Can you work these out from the model? Positions are in its coordinate system, mm. Face numbers are marked on the shaded views. A direction names the side the tool comes from. Give positions to 0.01 mm unless a question says otherwise; leave off trailing zeros. Write each loop counter-clockwise with the first axis right and the second up, starting at its lowest first coordinate (ties: lowest second). Pieces come first, ordered by that corner, then holes.
1. I'm going to push flat-ended pins straight in: pin 1 (4 mm diameter, centred on x = 215.5, z = -201, fed in from +Y); pin 2 (15 mm diameter, centred on x = 138.5, z = -123.5, fed in from +Y); pin 3 (4 mm diameter, centred on x = 149.5, y = 10, fed in from -Z); pin 4 (14.5 mm diameter, centred on x = 280.66, z = -260.34, fed in from -Y). Where does each tip first touch, or does it pass through?
2. If I drill on probe 1 along Z at (x, y) = (303, 29); probe 2 along Z at (x, y) = (373, 12); probe 3 along X at (y, z) = (5.5, -312), over which ranges is the centre line in solid material (lowest first)?
3. Suppose I cut it at D-D (x = 303.4). Please give me the cut outline in (y, z).
4. Suppose I cut it at A-A (x = 373). Please give me the cut outline in (y, z), and give its area (3 significant figures).
5. Suppose I cut it at C-C (z = -11). Please give me the cut outline in (x, y), and give its area (3 significant figures).
6. Thinking about a two-plate mould opening in X: for the marked faces 6, 7 and 8, which applies, pulls with the +X half, pulls with the -X half, needs draft (parallel to the pull), parting line crosses it, or undercut?
7. On a 3-axis mill with a long thin cutter (end or side, diameter ignored), from which of +Z, -Z, +X, -X, +Y, -Y can I reach the whole of each face in a straight line? I mean the marked faces 1, 2, 3, 4 and 5. Say none if no direction works.
8. Suppose I cut it at B-B (z = -274). Please give me the cut outline in (x, y).
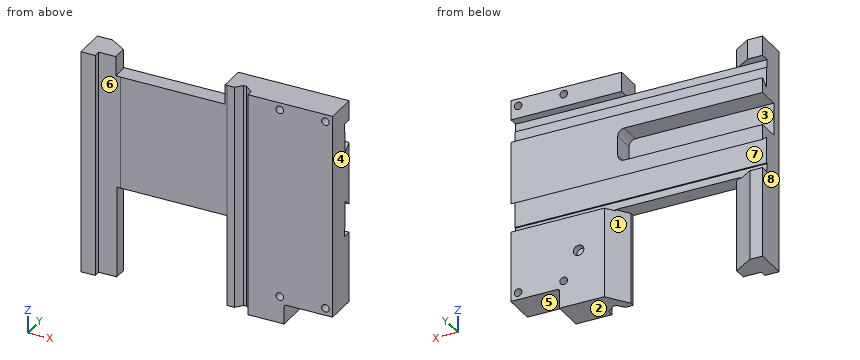
Autodesk Inventor part; units mm, degrees
ref_plane "YZ Plane" through (0, 0, 0) normal (1, 0, 0) x (0, 1, 0)
ref_plane "XZ Plane" through (0, 0, 0) normal (0, 1, 0) x (-1, 0, 0)
ref_plane "XY Plane" through (0, 0, 0) normal (0, 0, 1) x (1, 0, 0)
sketch "Sketch1" plane through (0, 0, 0) normal (0, 1, 0) x (-1, 0, 0)
  line L0 (0, 0) -> (-384, 0)
  line L1 (-384, 0) -> (-384, -343)
  line L2 (-384, -343) -> (0, -343)
  line L3 (0, -343) -> (0, 0)
  dimension "d0" = 384
  dimension "d1" = 343
extrude "Extrusion1" add sketch "Sketch1" along normal blind 48.5
sketch "Sketch3" plane through (384, 0, 0) normal (1, 0, 0) x (0, 0, -1)
  line L0 (0, 0) -> (343, 0)
  line L1 (0, 0) -> (0, 48.5)
  line L2 (343, 0) -> (343, 48.5)
  line L3 (30, 48.5) -> (65, 48.5)
  line L4 (30, 48.5) -> (30, 37)
  line L5 (65, 48.5) -> (74.6496, 37)
  line L6 (43, 37) -> (74.6496, 37)
  line L7 (30, 37) -> (30, 35)
  line L8 (30, 35) -> (43, 35)
  line L9 (43, 35) -> (43, 37)
  dimension "d23" = 35
  dimension "d37" = 2
  dimension "d38" = 13
extrude "Extrusion2" cut sketch "Sketch3" against normal through all
sketch "Sketch7" plane through (384, 0, 0) normal (1, 0, 0) x (0, 0, -1)
  line L0 (65, 48.5) -> (343, 48.5)
  line L1 (65, 48.5) -> (161, 48.5)
  line L2 (161, 48.5) -> (174.2196, 48.5) construction
  line L3 (161, 48.5) -> (205, 48.5)
  line L4 (0, 0) -> (343, 0)
  line L5 (151.3504, 37) -> (192, 37)
  line L6 (205, 37) -> (205, 48.5)
  line L7 (161, 48.5) -> (151.3504, 37)
  line L8 (161, 48.5) -> (183.0653, 48.5) construction
  line L9 (205, 37) -> (205, 35)
  line L10 (205, 35) -> (192, 35)
  line L11 (192, 35) -> (192, 37)
  dimension "d27" = 96
  dimension "d29" = 44
  dimension "d32" = 130
extrude "Extrusion3" cut sketch "Sketch7" against normal through all
sketch "Sketch8" plane through (0, 48.5, 0) normal (0, 1, 0) x (1, 0, 0)
  line L0 (310, 343) -> (310, 316)
  line L1 (313, 313) -> (384, 313)
  line L2 (384, 0) -> (384, 343)
  line L3 (384, 313) -> (384, 343)
  line L4 (384, 343) -> (310, 343)
  line L5 (384, 343) -> (0, 343)
  arc A0 (310, 316) -> (313, 313) centre (313, 316) ccw
  point P0 (0, 0)
  point P1 (310, 313)
  dimension "d43" = 30
  dimension "d46" = 3
extrude "Extrusion4" cut sketch "Sketch8" against normal through all
sketch "Sketch12" plane through (0, 48.5, 0) normal (0, 1, 0) x (1, 0, 0)
  line L0 (221, 113) -> (221, 128)
  line L1 (211, 88) -> (0, 88)
  line L2 (211, 138) -> (0, 138)
  arc A0 (211, 88) -> (221, 98) centre (211, 98) ccw
  arc A1 (221, 128) -> (211, 138) centre (211, 128) ccw
  line L3 (221, 98) -> (221, 113)
  line L4 (0, 88) -> (0, 138)
  point P0 (384, 161)
  point P1 (221, 88)
  dimension "d72" = 10
extrude "Extrusion8" cut sketch "Sketch12" against normal blind 33
sketch "Sketch28" plane through (0, 48.5, 0) normal (0, 1, 0) x (1, 0, 0)
  circle A0 centre (373, 302) radius 5.8
  circle A1 centre (303.4, 302) radius 5.8
  circle A2 centre (373, 11) radius 5.8
  circle A3 centre (303.4, 11) radius 5.8
  point P0 (0, 0)
  point P1 (384, 313)
  point P2 (384, 0)
  dimension "d146" = 11.6
  dimension "d149" = 11.6
  dimension "d152" = 11.6
  dimension "d155" = 11.6
extrude "Extrusion19" cut sketch "Sketch28" against normal through all
sketch "Sketch29" plane through (0, 48.5, 0) normal (0, 0, 1) x (1, 0, 0)
  line L0 (0, -48.5) -> (0, 0)
  line L1 (0, 0) -> (384, 0)
  line L2 (23, 0) -> (48, -16.2352)
  line L3 (23, 0) -> (48, -16.2352)
  line L4 (0, -48.5) -> (384, -48.5)
  line L5 (23, 0) -> (48, 0)
  line L6 (48, -16.2352) -> (48, 0)
  line L7 (384, -13.5) -> (0, -13.5)
  point P0 (48, -48.5)
  point P1 (215, -48.5)
  point P2 (20, -48.5)
extrude "Extrusion20" cut sketch "Sketch29" against normal up to surface (30 mm away) contours L7 L6 L2 | L2 L1 L6 L7
sketch "Sketch30" plane through (0, 0, 0) normal (0, 0, 1) x (1, 0, 0)
  line L0 (48, 48.5) -> (215, 48.5)
  line L1 (215, 48.5) -> (215, 0)
  line L2 (215, 0) -> (48, 0)
  line L3 (48, 0) -> (48, 48.5)
  point P0 (0, 0)
  point P1 (48, 0)
extrude "Extrusion21" cut sketch "Sketch30" against normal up to surface (30 mm away)
sketch "Sketch32" plane through (0, 48.5, 0) normal (0, 1, 0) x (1, 0, 0)
  line L0 (275, 266) -> (283, 266) construction
  circle A0 centre (280.6569, 260.3431) radius 8
  point P0 (0, 0)
  point P1 (255, 343)
  dimension "d168" = 16
extrude "Extrusion22" cut sketch "Sketch32" against normal blind 10
sketch "Sketch36" plane through (0, 0, -343) normal (0, 0, -1) x (-1, 0, 0)
  line L0 (-255, 0) -> (-243.6863, 11.3137)
  line L1 (-255, 0) -> (-239, 0) construction
  line L2 (-243.6863, 11.3137) -> (-239.0863, 11.3137)
  line L3 (-239.0863, 11.3137) -> (-229.7525, 1.9799)
  line L4 (-239.0863, 11.3137) -> (-225.8863, 11.3137) construction
  line L5 (-229.7525, 1.9799) -> (-217.7525, 1.9799)
  line L6 (-22, 0) -> (-22, 10)
  line L7 (-22, 10) -> (-55, 10)
  line L8 (-217.7525, 1.9799) -> (-217.7525, 0)
  line L9 (-55, 10) -> (-55, 0)
  line L10 (-255, 0) -> (-217.7525, 0)
  line L11 (-310, 0) -> (0, 0)
  line L12 (-55, 0) -> (-22, 0)
  dimension "d209" = 16
  dimension "d210" = 45
  dimension "d211" = 4.6
  dimension "d214" = 13.2
  dimension "d215" = 45
  dimension "d216" = 12
  dimension "d224" = 22
  dimension "d225" = 10
extrude "Extrusion23" cut sketch "Sketch36" against normal through all
sketch "Sketch37" plane through (0, 0, -343) normal (0, 0, -1) x (-1, 0, 0)
  line L0 (-217.7525, 1.9799) -> (-217.7525, 15.9799)
  line L1 (-217.7525, 15.9799) -> (-241.3863, 48.5)
  line L2 (-241.3863, 48.5) -> (-19.5919, 48.5)
  line L3 (-211, 48.5) -> (0, 48.5)
  line L4 (-48, 10) -> (-55, 10)
  line L5 (-217.7525, 0) -> (-217.7525, 1.9799)
  line L6 (-217.7525, 1.9799) -> (-217.7525, 0)
  line L7 (-215, 0) -> (-55, 0)
  line L8 (-217.7525, 0) -> (-55, 0)
  line L9 (-55, 10) -> (-55, 0)
  line L10 (-55, 0) -> (-55, 10)
  line L11 (-217.7525, 15.9799) -> (-49.7525, 15.9799) construction
  line L12 (-55, 10) -> (-49.7525, 10)
  line L13 (-49.7525, 10) -> (-49.7525, 29)
  line L14 (-49.7525, 29) -> (-19.5919, 48.5)
  line L15 (0, 48.5) -> (-23, 48.5)
  point P0 (0, 0)
  dimension "d229" = 14
  dimension "d232" = 19
extrude "Extrusion24" cut sketch "Sketch37" against normal blind 140
sketch "Sketch38" plane through (0, 0, -203) normal (0, 0, -1) x (-1, 0, 0)
  line L0 (-49.7525, 29) -> (-49.7525, 10)
  line L1 (-55, 9.9841) -> (-217.7525, 9.4921)
  line L2 (-217.7525, 1.9799) -> (-217.7525, 15.9799)
  line L3 (-217.7525, 0) -> (-217.7525, 1.9799)
  line L4 (-217.7525, 9.4921) -> (-217.7525, 0)
  line L5 (-215, 0) -> (-55, 0)
  line L6 (-217.7525, 0) -> (-55, 0)
  line L7 (-55, 10) -> (-55, 0)
  line L8 (-55, 0) -> (-55, 10)
  line L9 (-55, 10) -> (-55, 0)
  point P0 (0, 0)
extrude "Extrusion25" cut sketch "Sketch38" against normal through all
sketch "Sketch40" plane through (0, 0, -343) normal (0, 0, -1) x (-1, 0, 0)
  line L0 (-229.5482, 9.4921) -> (-238.1559, 19.4995)
  line L1 (-229.5482, 9.4921) -> (-216.3482, 9.4921) construction
  line L2 (-238.1559, 19.4995) -> (-242.7559, 19.4995)
  line L3 (-242.7559, 19.4995) -> (-255, 9.1999)
  line L4 (-242.7559, 19.4995) -> (-226.7559, 19.4995) construction
  line L5 (-243.6863, 11.3137) -> (-255, 0)
  line L6 (-255, 9.1999) -> (-255, 0)
  line L7 (-229.5482, 9.4921) -> (-217.7525, 9.4921)
  line L8 (-217.7525, 9.4921) -> (-217.7525, 1.9799)
  line L9 (-217.7525, 9.4921) -> (-217.7525, 1.9799)
  line L10 (-217.7525, 1.9799) -> (-217.7525, 9.4921)
  line L11 (-217.7525, 1.9799) -> (-229.7525, 1.9799)
  line L12 (-229.7525, 1.9799) -> (-239.0863, 11.3137)
  line L13 (-229.7525, 1.9799) -> (-239.0863, 11.3137)
  line L14 (-239.0863, 11.3137) -> (-243.6863, 11.3137)
  line L15 (-255, 0) -> (-243.6863, 11.3137)
  dimension "d240" = 13.2
  dimension "d242" = 4.6
  dimension "d243" = 16
extrude "Extrusion26" cut sketch "Sketch40" against normal through all
properties part number "saddle" material "Iron, Cast"
Checks:
1. pin 1: stops at y = 35
1. pin 2: stops at y = 15.5
1. pin 3: stops at z = -203
1. pin 4: stops at y = 0
2. probe 1: z = -343 to -307.79, -296.21 to -16.79, -5.21 to 0
2. probe 2: z = -313 to -307.8, -296.2 to -16.8, -5.2 to 0
2. probe 3: x = 0 to 22, 255 to 384
3. outline: (0, -343) - (48.5, -343) - (48.5, -307.8) - (0, -307.8) - close; (0, -296.2) - (48.5, -296.2) - (48.5, -205) - (35, -205) - (35, -192) - (37, -192) - (37, -151.35) - (48.5, -161) - (48.5, -65) - (37, -74.65) - (37, -43) - (35, -43) - (35, -30) - (48.5, -30) - (48.5, -16.8) - (0, -16.8) - close; (0, -5.2) - (48.5, -5.2) - (48.5, 0) - (0, 0) - close
4. outline: (0, -313) - (48.5, -313) - (48.5, -307.8) - (0, -307.8) - close; (0, -296.2) - (48.5, -296.2) - (48.5, -205) - (35, -205) - (35, -192) - (37, -192) - (37, -151.35) - (48.5, -161) - (48.5, -65) - (37, -74.65) - (37, -43) - (35, -43) - (35, -30) - (48.5, -30) - (48.5, -16.8) - (0, -16.8) - close; (0, -5.2) - (48.5, -5.2) - (48.5, 0) - (0, 0) - close
4. area: 13,000 mm2
5. outline: (0, 0) - (22, 0) - (22, 10) - (48, 10) - (48, 32.26) - (23, 48.5) - (0, 48.5) - close; (215, 9.5) - (217.75, 9.49) - (229.55, 9.49) - (238.16, 19.5) - (242.76, 19.5) - (255, 9.2) - (255, 0) - (297.6, 0) - (297.6, 48.5) - (215, 48.5) - close; (309.2, 0) - (367.2, 0) - (367.2, 48.5) - (309.2, 48.5) - close; (378.8, 0) - (384, 0) - (384, 48.5) - (378.8, 48.5) - close
5. area: 8,410 mm2
6. face 6: undercut
6. face 7: needs draft
6. face 8: pulls with the -X half
7. face 1: -Z, +Y
7. face 2: -Z, +X, -X, +Y, -Y
7. face 3: -X, +Y
7. face 4: +Z, -Z, +X, +Y, -Y
7. face 5: -Z, +X, +Y, -Y
8. outline: (0, 0) - (22, 0) - (22, 10) - (49.75, 10) - (49.75, 29) - (19.59, 48.5) - (0, 48.5) - close; (217.75, 9.49) - (229.55, 9.49) - (238.16, 19.5) - (242.76, 19.5) - (255, 9.2) - (255, 0) - (384, 0) - (384, 48.5) - (241.39, 48.5) - (217.75, 15.98) - close
